Geometry check sheet. Reference: the model listing, model coordinates, mm. A direction names the side the tool comes from. Round coordinates to 2 decimals unless told otherwise and drop trailing zeros. Order: outer loops, then holes, each group sorted by start corner. A loop starts at its lowest first (then second) coordinate and runs counter-clockwise, first axis right, second up. Notation, with made-up numbers: (-8.75, 10.5) - (25.25, 10.5) arc R21 cw to (25.25, 30.5) - close; hole circle Ø6 at (-21, 28). An arc over 180 degrees is marked (long way). Write each question's results on one line, items separated by ' | '.
Autodesk Inventor part; units mm, degrees
ref_plane "YZ Plane" through (0, 0, 0) normal (1, 0, 0) x (0, 1, 0)
ref_plane "XZ Plane" through (0, 0, 0) normal (0, 1, 0) x (-1, 0, 0)
ref_plane "XY Plane" through (0, 0, 0) normal (0, 0, 1) x (1, 0, 0)
sketch "スケッチ1" plane through (0, 0, 0) normal (0, 0, 1) x (1, 0, 0)
  line L0 (-11.3154, 7.0975) -> (3.6846, 7.0975)
  line L1 (3.6846, 7.0975) -> (3.6846, -22.9025)
  line L2 (3.6846, -22.9025) -> (-11.3154, -22.9025)
  line L3 (-11.3154, -22.9025) -> (-11.3154, 7.0975)
  point P0 (0, 0)
  dimension "d0" = 15
  dimension "d1" = 30
extrude "押し出し1" add sketch "スケッチ1" along normal blind 330
sketch "スケッチ2" plane through (3.6846, -22.9025, 0) normal (1, 0, 0) x (0, 0, -1)
  circle A0 centre (-320, 15) radius 1.5
  line L0 (0, 30) -> (-330, 30)
  line L1 (-330, 0) -> (-330, 30)
  circle A1 centre (-310, 15) radius 1.5
  circle A2 centre (-300, 15) radius 1.5
  circle A3 centre (-30, 15) radius 1.5
  circle A4 centre (-20, 15) radius 1.5
  circle A5 centre (-10, 15) radius 1.5
  line L2 (0, 30) -> (0, 0)
  point P0 (0, 22.9025)
  dimension "d4" = 3
  dimension "d5" = 15
  dimension "d6" = 10
  dimension "d7" = 3
  dimension "d8" = 3
  dimension "d9" = 3
  dimension "d10" = 3
  dimension "d11" = 3
  dimension "d12" = 10
  dimension "d13" = 10
  dimension "d14" = 10
  dimension "d15" = 10
  dimension "d16" = 10
hole "穴1" at (3.6846, -7.9025, 320) at (3.6846, -7.9025, 310) at (3.6846, -7.9025, 300) at (3.6846, -7.9025, 10) at (3.6846, -7.9025, 20) at (3.6846, -7.9025, 30) direction (-1, 0, 0) diameter 3 depth 15
sketch "スケッチ3" plane through (-11.3154, 7.0975, 0) normal (0, 1, 0) x (1, 0, 0)
  circle A0 centre (7.5, -15) radius 1.5
  line L0 (0, 0) -> (15, 0)
  circle A1 centre (7.5, -25) radius 1.5
  circle A2 centre (7.5, -35) radius 1.5
  circle A3 centre (7.5, -315) radius 1.5
  line L1 (15, -330) -> (0, -330)
  circle A4 centre (7.5, -305) radius 1.5
  circle A5 centre (7.5, -295) radius 1.5
  point P0 (11.3154, 0)
  dimension "d24" = 3
  dimension "d25" = 15
  dimension "d26" = 3
  dimension "d27" = 3
  dimension "d28" = 3
  dimension "d29" = 15
  dimension "d30" = 3
  dimension "d31" = 3
  dimension "d32" = 10
  dimension "d33" = 10
  dimension "d34" = 10
  dimension "d35" = 10
hole "穴2" at (-3.8154, 7.0975, 295) at (-3.8154, 7.0975, 305) at (-3.8154, 7.0975, 315) at (-3.8154, 7.0975, 15) at (-3.8154, 7.0975, 25) at (-3.8154, 7.0975, 35) direction (0, -1, 0) diameter 3 depth 30
sketch "スケッチ4" plane through (0, 0, 330) normal (0, 0, 1) x (1, 0, 0)
  line L0 (-9.8154, 5.5975) -> (2.1846, 5.5975)
  line L1 (2.1846, 5.5975) -> (2.1846, -21.4025)
  line L2 (2.1846, -21.4025) -> (-9.8154, -21.4025)
  line L3 (-9.8154, -21.4025) -> (-9.8154, 5.5975)
  line L4 (3.6846, 7.0975) -> (-11.3154, 7.0975)
  line L5 (-11.3154, 7.0975) -> (-11.3154, -22.9025)
  point P0 (0, 0)
  dimension "d43" = 12
  dimension "d44" = 27
  dimension "d45" = 1.5
  dimension "d46" = 1.5
extrude "押し出し2" cut sketch "スケッチ4" against normal blind 330
sketch "スケッチ5" plane through (3.6846, -22.9025, 0) normal (1, 0, 0) x (0, 0, -1)
  circle A0 centre (-141, 15) radius 1.5
  line L0 (0, 30) -> (-330, 30)
  line L1 (0, 30) -> (0, 0)
  point P0 (0, 22.9025)
  dimension "d49" = 3
  dimension "d50" = 15
  dimension "d51" = 141
hole "穴3" at (3.6846, -7.9025, 141) direction (-1, 0, 0) diameter 3 depth 15
equation "\"BendRadius\" = Thickness"
equation "\"BendReliefWidth\" = Thickness"
equation "\"BendReliefDepth\" = 0.5 * Thickness"
equation "\"CornerReliefSize\" = 4 * Thickness"
equation "\"MinimumRemnant\" = 2 * Thickness"
equation "\"TransitionRadius\" = BendRadius"
equation "\"JacobiRadiusSize\" = BendRadius"
equation "\"GapSize\" = Thickness"
properties part number "nhk17" material "アルミニウム 6061"
(1) Section check A-A (y = -12.5). Record the cut outline in (x, z), then the cut area to 3 significant figures.
Answers follow:
outline: (-11.32, 0) - (-9.82, 0) - (-9.82, 330) - (-11.32, 330) - close; (2.18, 0) - (3.68, 0) - (3.68, 330) - (2.18, 330) - close | area: 990 mm²
(2) Access from +Z, -Z, +X, -X, +Y, -Y to the whole of each face (thin tool, end or side, straight path). Record for faces 1 (the face through (-4, 7.098, 163)), 2 (the face through (2.185, -8, 167)).
Answers follow:
face 1: +Z, -Z, +X, -X, +Y | face 2: +Z, -Z
(3) Draft check along X on faces 3 (the face through (-4, 5.598, 167)), 4 (the face through (-11.315, -8, 163)), 5 (the face through (3.685, -8, 163)), 6 (the face through (-10, -7, 330)). Enter one of: released by +X, released by -X, zero draft, split by the parting line, or undercut.
Answers follow:
face 3: undercut | face 4: released by -X | face 5: released by +X | face 6: zero draft
(4) Material ranges on line 1 (X direction, y = -16.25, z = 150); line 2 (X direction, y = -21.9, z = 295); line 3 (Y direction, x = -0.75, z = 17.5), recorded low to high.
Answers follow:
line 1: -11.32 to -9.82, 2.18 to 3.68 | line 2: -11.32 to -5.32, -2.32 to 3.68 | line 3: -22.9 to -21.4, 5.6 to 7.1
(5) Section check B-B (z = 159.5). Record the cut outline in (x, y), then the cut area to 3 significant figures.
Answers follow:
outline: (-11.32, -22.9) - (3.68, -22.9) - (3.68, 7.1) - (-11.32, 7.1) - close; hole (-9.82, -21.4) - (2.18, -21.4) - (2.18, 5.6) - (-9.82, 5.6) - close | area: 126 mm²
